For this review, use the dimensioned drawing (mm, ordinates from the lowest corner) and the shaded views. A direction names the side the tool comes from. Coordinates: 2 decimals unless noted, no trailing zeros. Write each loop counter-clockwise with the first axis right and the second up, starting at its lowest first coordinate (ties: lowest second). Pieces come first, ordered by that corner, then holes.
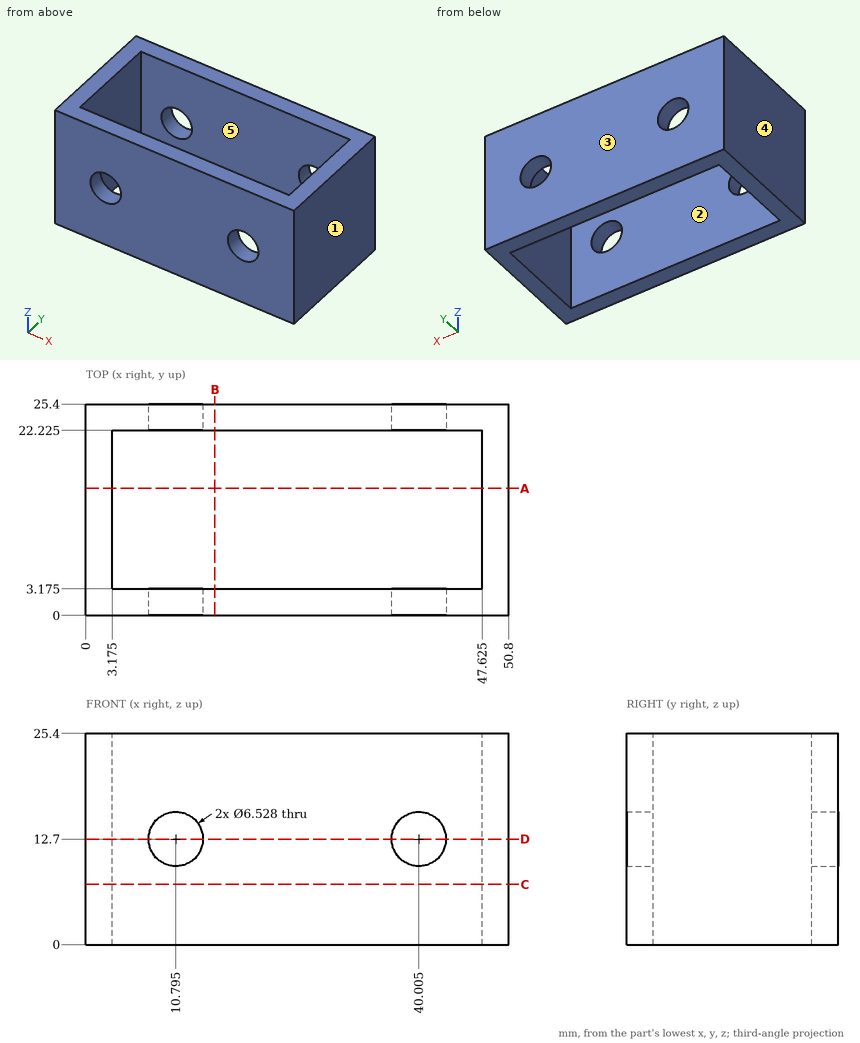
(1) Wall thickness on line 1 (X direction, y = 23.35, z = 12.7); line 2 (Y direction, x = 16, z = 13.5) (3 decimals); line 3 (X direction, y = 23.25, z = 10.25): over which ranges is each line inside the solid? List them lowest first.
(2) Mouldability with a two-part tool opening along Y and no side actions: class the marked faces 1, 2 and 3 as +Y half, -Y half, draft (parallel to the pull), parting line (faces both ways), or undercut.
(3) Consider section D-D (z = 12.7). Give the boundary of the cut face in (x, y) (1 decimal), plus the area to 3 significant figures.
(4) Consider section A-A (y = 15.25). Give the boundary of the cut face in (x, z) (3 decimals), plus the area to 3 significant figures.
(5) Consider section B-B (x = 15.5). Give the boundary of the cut face in (y, z) (3 decimals), plus the area to 3 significant figures.
(6) Consider section C-C (z = 7.25). Give the boundary of the cut face in (x, y) (3 decimals).
(7) For the marked faces 4 and 5, list the 3-axis set-ups (+Z, -Z, +X, -X, +Y, -Y) from which the entire face can be reached by the end or side of a thin tool; tool diameter is ignored.
Results:
1. line 1: x = 0 to 7.53, 14.06 to 36.74, 43.27 to 50.8
1. line 2: y = 0 to 3.175, 22.225 to 25.4
1. line 3: x = 0 to 8.64, 12.95 to 37.85, 42.16 to 50.8
2. face 1: draft
2. face 2: undercut
2. face 3: +Y half
3. outline: (0, 0) - (7.5, 0) - (7.5, 3.2) - (3.2, 3.2) - (3.2, 22.2) - (7.5, 22.2) - (7.5, 25.4) - (0, 25.4) - close; (14.1, 0) - (36.7, 0) - (36.7, 3.2) - (14.1, 3.2) - close; (14.1, 22.2) - (36.7, 22.2) - (36.7, 25.4) - (14.1, 25.4) - close; (43.3, 0) - (50.8, 0) - (50.8, 25.4) - (43.3, 25.4) - (43.3, 22.2) - (47.6, 22.2) - (47.6, 3.2) - (43.3, 3.2) - close
3. area: 361 mm2
4. outline: (0, 0) - (3.175, 0) - (3.175, 25.4) - (0, 25.4) - close; (47.625, 0) - (50.8, 0) - (50.8, 25.4) - (47.625, 25.4) - close
4. area: 161 mm2
5. outline: (0, 0) - (3.175, 0) - (3.175, 25.4) - (0, 25.4) - close; (22.225, 0) - (25.4, 0) - (25.4, 25.4) - (22.225, 25.4) - close
5. area: 161 mm2
6. outline: (0, 0) - (50.8, 0) - (50.8, 25.4) - (0, 25.4) - close; hole (3.175, 3.175) - (47.625, 3.175) - (47.625, 22.225) - (3.175, 22.225) - close
7. face 4: +Z, -Z, -X, +Y, -Y
7. face 5: +Z, -Z
